Build history of the part. All positions in model axes, mm. A direction names the side the tool comes from. Give positions to 0.01 mm unless a question says otherwise; leave off trailing zeros. Loops run counter-clockwise (first coordinate to the right, second up) from the corner with the lowest first, then second, coordinate; pieces in that order, holes last. Notation, with made-up numbers: M 36,-24.75 L 87,-24.75 A17 ccw 87,-19.75 Z; hole C 16,45.25 d10. An arc over 180 degrees is marked long. Answer in a Markdown table with one row per item. Add a question column.
```python
from build123d import *

# Parameters (mm, degrees)
F1_W     = 53.687666
F1_H     = 59.399114
F1_R     = 15.376156
F2_DEPTH = 25.4
F3_DEPTH = 60.706
F4_R     = 13.987853
F5_DEPTH = 95.25


with BuildPart() as f2:
    # F1 (on face) → F2 (new body)
    with BuildSketch(Plane.XY):
        Rectangle(F1_W, F1_H)
        Circle(F1_R, mode=Mode.SUBTRACT)
    extrude(amount=F2_DEPTH)

    # F1 (on face) → F3 (join)
    with BuildSketch(Plane.XY):
        Circle(F1_R)
    extrude(amount=F3_DEPTH)

    # F4 (on face) → F5 (cut)
    with BuildSketch(Plane.XY.offset(60.706)):
        Circle(F4_R)
    extrude(amount=-F5_DEPTH, mode=Mode.SUBTRACT)


solid = f2.part
```
(1) Slice it at A-A, the plane x = 0. Give the cut face in (y, z), then the cut area to 3 significant figures.
(2) Wall check: line 1 (Y direction, x = 0, z = 15.5); line 2 (Y direction, x = 0, z = 45); line 3 (Z direction, x = -18, y = -23). Give the ranges that are in metal, low to high.
(3) Slice it at C-C, the plane z = 4.5. Give the cut face in (x, y), then the cut area to 3 significant figures.
(4) Pin check, flat tips, straight feed: pin 1 (25 mm diameter, centred on x = 0, y = 0, fed in from -Z); pin 2 (2 mm diameter, centred on y = -14.5, z = 34.5, fed in from -X); pin 3 (8 mm diameter, centred on x = 14, y = -23, fed in from -Z); pin 4 (1.5 mm diameter, centred on y = 1, z = 44, fed in from +X). Stop position of each tip, or through.
(5) Slice it at D-D, the plane x = -17. Give the cut face in (y, z), then the cut area to 3 significant figures.
(6) Tool access for faces 1 (the cylindrical face through (8.266, 12.965, 42.806)), 2 (the flat face through (3, -14, 60.706)): list every direction of +Z, -Z, +X, -X, +Y, -Y with a clear straight run to the whole face (end or side of a thin tool).
(7) Slice it at B-B, the plane y = 0. Give the cut face in (x, z), then the cut area to 3 significant figures.
Solution:
| question | item | result |
|---|---|---|
| 1 | outline | M -29.7,0 L -13.99,0 L -13.99,60.71 L -15.38,60.71 L -15.38,25.4 L -29.7,25.4 Z; M 13.99,0 L 29.7,0 L 29.7,25.4 L 15.38,25.4 L 15.38,60.71 L 13.99,60.71 Z |
| 1 | area | 896 mm^2 |
| 2 | line 1 | -29.7 to -13.99, 13.99 to 29.7 |
| 2 | line 2 | -15.38 to -13.99, 13.99 to 15.38 |
| 2 | line 3 | 0 to 25.4 |
| 3 | outline | M -26.84,-29.7 L 26.84,-29.7 L 26.84,29.7 L -26.84,29.7 Z; hole C 0,0 d27.98 |
| 3 | area | 2,570 mm^2 |
| 4 | pin 1 | through |
| 4 | pin 2 | x = -7.36 |
| 4 | pin 3 | z = 0 |
| 4 | pin 4 | x = 15.37 |
| 5 | outline | M -29.7,0 L 29.7,0 L 29.7,25.4 L -29.7,25.4 Z |
| 5 | area | 1,510 mm^2 |
| 6 | face 1 | +Z |
| 6 | face 2 | +Z, +X, -X, +Y, -Y |
| 7 | outline | M -26.84,0 L -13.99,0 L -13.99,60.71 L -15.38,60.71 L -15.38,25.4 L -26.84,25.4 Z; M 13.99,0 L 26.84,0 L 26.84,25.4 L 15.38,25.4 L 15.38,60.71 L 13.99,60.71 Z |
| 7 | area | 751 mm^2 |
